from build123d import *

# Parameters (mm, degrees)
BOX017_W               = 5
BOX017_H               = 32.5
BOX017_DEPTH           = 5
BOX017_PITCH_ANGLE     = 45
BOX016_W               = 3
BOX016_H               = 32.5
BOX016_DEPTH           = 15
CYLINDER001_R          = 1.6
CYLINDER001_DEPTH      = 35
CYLINDER001_ROLL_ANGLE = 90
CYLINDER_R             = 1.6
CYLINDER_DEPTH         = 10
BOX006_W               = 10
BOX006_H               = 32.5
BOX006_DEPTH           = 10
BOX006_PITCH_ANGLE     = -10
BOX001_W               = 35
BOX001_H               = 32.5
BOX001_DEPTH           = 3
BOX002_W               = 35
BOX002_H               = 3
BOX002_DEPTH           = 3
BOX003_W               = 35
BOX003_H               = 3
BOX003_DEPTH           = 3
BOX004_W               = 35
BOX004_H               = 3
BOX004_DEPTH           = 3
BOX005_W               = 35
BOX005_H               = 3
BOX005_DEPTH           = 3
BOX007_W               = 9
BOX007_H               = 32.5
BOX007_DEPTH           = 13.5
BOX008_W               = 3
BOX008_H               = 3
BOX008_DEPTH           = 52
BOX009_W               = 3
BOX009_H               = 3
BOX009_DEPTH           = 52
BOX010_W               = 3
BOX010_H               = 3
BOX010_DEPTH           = 52
BOX011_W               = 3
BOX011_H               = 3
BOX011_DEPTH           = 52
BOX012_W               = 3
BOX012_H               = 32.5
BOX012_DEPTH           = 6.5
BOX013_W               = 30
BOX013_H               = 32.5
BOX013_DEPTH           = 3
BOX014_W               = 30
BOX014_H               = 3
BOX014_DEPTH           = 3
BOX015_W               = 30
BOX015_H               = 3
BOX015_DEPTH           = 3
BOX_W                  = 3
BOX_H                  = 32.5
BOX_DEPTH              = 42.5


with BuildPart() as cube017:
    # Box017 → Box017 (new body)
    with BuildSketch(Plane.XY):
        with Locations((2.5, 16.25)):
            Rectangle(BOX017_W, BOX017_H)
    extrude(amount=BOX017_DEPTH)


with BuildPart() as cube017_1:
    # Box017 pitch: moved
    add(cube017.part.rotate(Axis((0, 0, 0), (0, 1, 0)), BOX017_PITCH_ANGLE))


with BuildPart() as cube017_2:
    # Box017 placement: moved
    add(cube017_1.part.moved(Location((0, 0, 0.5))))


with BuildPart() as cube016:
    # Box016 → Box016 (new body)
    with BuildSketch(Plane.XY.offset(-14.5)):
        with Locations((1.5, 16.25)):
            Rectangle(BOX016_W, BOX016_H)
    extrude(amount=BOX016_DEPTH)


with BuildPart() as cylinder001:
    # Cylinder001 → Cylinder001 (new body)
    with BuildSketch(Plane.XY):
        Circle(CYLINDER001_R)
    extrude(amount=CYLINDER001_DEPTH)


with BuildPart() as cylinder001_1:
    # Cylinder001 roll: moved
    add(cylinder001.part.rotate(Axis((0, 0, 0), (1, 0, 0)), CYLINDER001_ROLL_ANGLE))


with BuildPart() as cylinder001_2:
    # Cylinder001 placement: moved
    add(cylinder001_1.part.moved(Location((-1.5, 33, 5))))


with BuildPart() as cylinder:
    # Cylinder → Cylinder (new body)
    with BuildSketch(Plane(origin=(-19, 16.25, -8), x_dir=(1, 0, 0), z_dir=(0, 0, 1))):
        Circle(CYLINDER_R)
    extrude(amount=CYLINDER_DEPTH)


with BuildPart() as cube006:
    # Box006 → Box006 (new body)
    with BuildSketch(Plane.XY):
        with Locations((5, 16.25)):
            Rectangle(BOX006_W, BOX006_H)
    extrude(amount=BOX006_DEPTH)


with BuildPart() as cube006_1:
    # Box006 pitch: moved
    add(cube006.part.rotate(Axis((0, 0, 0), (0, 1, 0)), BOX006_PITCH_ANGLE))


with BuildPart() as cube006_2:
    # Box006 placement: moved
    add(cube006_1.part.moved(Location((29, 0, 32))))


with BuildPart() as cube001:
    # Box001 → Box001 (new body)
    with BuildSketch(Plane.XY.offset(42.5)):
        with Locations((17.5, 16.25)):
            Rectangle(BOX001_W, BOX001_H)
    extrude(amount=BOX001_DEPTH)


with BuildPart() as cube002:
    # Box002 → Box002 (new body)
    with BuildSketch(Plane.XY.offset(45.5)):
        with Locations((17.5, 1.5)):
            Rectangle(BOX002_W, BOX002_H)
    extrude(amount=BOX002_DEPTH)


with BuildPart() as cube003:
    # Box003 → Box003 (new body)
    with BuildSketch(Plane(origin=(0, 29.5, 45.5), x_dir=(1, 0, 0), z_dir=(0, 0, 1))):
        with Locations((17.5, 1.5)):
            Rectangle(BOX003_W, BOX003_H)
    extrude(amount=BOX003_DEPTH)


with BuildPart() as cube004:
    # Box004 → Box004 (new body)
    with BuildSketch(Plane(origin=(0, 10, 45.5), x_dir=(1, 0, 0), z_dir=(0, 0, 1))):
        with Locations((17.5, 1.5)):
            Rectangle(BOX004_W, BOX004_H)
    extrude(amount=BOX004_DEPTH)


with BuildPart() as cube005:
    # Box005 → Box005 (new body)
    with BuildSketch(Plane(origin=(0, 19.5, 45.5), x_dir=(1, 0, 0), z_dir=(0, 0, 1))):
        with Locations((17.5, 1.5)):
            Rectangle(BOX005_W, BOX005_H)
    extrude(amount=BOX005_DEPTH)


with BuildPart() as cube007:
    # Box007 → Box007 (new body)
    with BuildSketch(Plane(origin=(-6, 0, -4), x_dir=(1, 0, 0), z_dir=(0, 0, 1))):
        with Locations((4.5, 16.25)):
            Rectangle(BOX007_W, BOX007_H)
    extrude(amount=BOX007_DEPTH)


with BuildPart() as cube008:
    # Box008 → Box008 (new body)
    with BuildSketch(Plane(origin=(-3, 0, -3.5), x_dir=(1, 0, 0), z_dir=(0, 0, 1))):
        with Locations((1.5, 1.5)):
            Rectangle(BOX008_W, BOX008_H)
    extrude(amount=BOX008_DEPTH)


with BuildPart() as cube009:
    # Box009 → Box009 (new body)
    with BuildSketch(Plane(origin=(-3, 29.5, -3.5), x_dir=(1, 0, 0), z_dir=(0, 0, 1))):
        with Locations((1.5, 1.5)):
            Rectangle(BOX009_W, BOX009_H)
    extrude(amount=BOX009_DEPTH)


with BuildPart() as cube010:
    # Box010 → Box010 (new body)
    with BuildSketch(Plane(origin=(-3, 19.5, -3.5), x_dir=(1, 0, 0), z_dir=(0, 0, 1))):
        with Locations((1.5, 1.5)):
            Rectangle(BOX010_W, BOX010_H)
    extrude(amount=BOX010_DEPTH)


with BuildPart() as cube011:
    # Box011 → Box011 (new body)
    with BuildSketch(Plane(origin=(-3, 10, -3.5), x_dir=(1, 0, 0), z_dir=(0, 0, 1))):
        with Locations((1.5, 1.5)):
            Rectangle(BOX011_W, BOX011_H)
    extrude(amount=BOX011_DEPTH)


with BuildPart() as cube012:
    # Box012 → Box012 (new body)
    with BuildSketch(Plane.XY.offset(-6.5)):
        with Locations((1.5, 16.25)):
            Rectangle(BOX012_W, BOX012_H)
    extrude(amount=BOX012_DEPTH)


with BuildPart() as cube013:
    # Box013 → Box013 (new body)
    with BuildSketch(Plane(origin=(-30, 0, -7), x_dir=(1, 0, 0), z_dir=(0, 0, 1))):
        with Locations((15, 16.25)):
            Rectangle(BOX013_W, BOX013_H)
    extrude(amount=BOX013_DEPTH)


with BuildPart() as cube014:
    # Box014 → Box014 (new body)
    with BuildSketch(Plane(origin=(-30, 0, -10), x_dir=(1, 0, 0), z_dir=(0, 0, 1))):
        with Locations((15, 1.5)):
            Rectangle(BOX014_W, BOX014_H)
    extrude(amount=BOX014_DEPTH)


with BuildPart() as cube015:
    # Box015 → Box015 (new body)
    with BuildSketch(Plane(origin=(-30, 29.5, -10), x_dir=(1, 0, 0), z_dir=(0, 0, 1))):
        with Locations((15, 1.5)):
            Rectangle(BOX015_W, BOX015_H)
    extrude(amount=BOX015_DEPTH)


with BuildPart() as cut004:
    # Box → Box (new body)
    with BuildSketch(Plane.XY):
        with Locations((1.5, 16.25)):
            Rectangle(BOX_W, BOX_H)
    extrude(amount=BOX_DEPTH)

    # Fusion: union Cube001, Cube002, Cube003, Cube004, Cube005, Cube007, Cube008, Cube009, Cube010, Cube011, Cube012, Cube013, Cube014, Cube015
    add(cube001.part)
    add(cube002.part)
    add(cube003.part)
    add(cube004.part)
    add(cube005.part)
    add(cube007.part)
    add(cube008.part)
    add(cube009.part)
    add(cube010.part)
    add(cube011.part)
    add(cube012.part)
    add(cube013.part)
    add(cube014.part)
    add(cube015.part)

    # Cut: cut Cube006
    add(cube006_2.part, mode=Mode.SUBTRACT)

    # Cut001: cut Cylinder
    add(cylinder.part, mode=Mode.SUBTRACT)

    # Cut002: cut Cylinder001
    add(cylinder001_2.part, mode=Mode.SUBTRACT)

    # Cut003: cut Cube016
    add(cube016.part, mode=Mode.SUBTRACT)

    # Cut004: cut Cube017
    add(cube017_2.part, mode=Mode.SUBTRACT)


solid = cut004.part
Could you check a few things on this model? Use its own coordinates, in mm. A direction names the side the tool comes from. Give positions to 0.01 mm unless a question says otherwise; leave off trailing zeros. Order: outer loops, then holes, each group sorted by start corner. A loop starts at its lowest first (then second) coordinate and runs counter-clockwise, first axis right, second up. Notation, with made-up numbers: (26.5, 66) -> (73.5, 66) arc R11 cw to (73.5, 81) -> close; hole circle Ø1 at (20, -39.75). An arc over 180 degrees is marked (long way). Answer in a Markdown table with one row per item. Add a question column.
Item 1: For faces 3 (the flat face through (-16, 16, -4)), 4 (the flat face through (0, 6, 27)), 5 (the flat face through (-15, 3, -9)), 6 (the flat face through (0, 16, -4)), which set-ups out of +Z, -Z, +X, -X, +Y, -Y let a thin tool reach every point of the face, with its end or its side?
Item 2: Imagine slicing it at B-B (y = 16.25). List the corners of the cut face in (x, z) for me.
Item 3: Please list where these lines run through material, in increasing order: probe 1 along Y at (x, z) = (-1.5, 31); probe 2 along Y at (x, z) = (-19, -5); probe 3 along X at (y, z) = (30.5, 5).
Item 4: We'd pull the mould along Y, two halves only. Please class faces 1 (the flat face through (1.5, 16, 2)), 2 (the flat face through (-1, 13, 38)): pulls with the +Y half, pulls with the -Y half, needs draft (parallel to the pull), parting line crosses it, or undercut.
Item 5: Imagine slicing it at A-A (x = -1.5). List the corners of the cut face in (y, z) for me, and give its area (3 significant figures).
Item 6: I'm going to push flat-ended pins straight in: P1, Ø4, axis at y = 23.5, z = 4, coming from the -X side; P2, Ø1.5, axis at y = 27, z = 13.5, coming from the -X side; P3, Ø1.9, axis at x = -19, y = 16.25, coming from the +Z side; P4, Ø8, axis at y = 14.5, z = 29, coming from the -X side. Where does each tip first touch, or does it pass through?
Item 7: Imagine slicing it at C-C (z = 5). List the corners of the cut face in (x, y) for me.
Item 8: Imagine slicing it at D-D (y = 25). List the corners of the cut face in (x, z) for me.
Result:
| question | item | result |
|---|---|---|
| 1 | face 3 | +Z, -X, +Y, -Y |
| 1 | face 4 | +Z, -X |
| 1 | face 5 | -Z, +X, -X |
| 1 | face 6 | -Z, +X, +Y, -Y |
| 2 | outline | (-30, -7) -> (-20.6, -7) -> (-20.6, -4) -> (-30, -4) -> close; (-17.4, -7) -> (0, -7) -> (0, 0.5) -> (3, 3.5) -> (3, 42.5) -> (30.96, 42.5) -> (35, 43.21) -> (35, 45.5) -> (0, 45.5) -> (0, 9.5) -> (-6, 9.5) -> (-6, -4) -> (-17.4, -4) -> close; hole circle Ø3.2 at (-1.5, 5) |
| 3 | probe 1 | 0 to 3, 10 to 13, 19.5 to 22.5, 29.5 to 32.5 |
| 3 | probe 2 | 0 to 14.65, 17.85 to 32.5 |
| 3 | probe 3 | -6 to -3.1, 0.1 to 3 |
| 4 | face 1 | needs draft |
| 4 | face 2 | undercut |
| 5 | outline | (0, -10) -> (3, -10) -> (3, -7) -> (29.5, -7) -> (29.5, -10) -> (32.5, -10) -> (32.5, 3.4) -> (0, 3.4) -> close; (0, 6.6) -> (32.5, 6.6) -> (32.5, 48.5) -> (29.5, 48.5) -> (29.5, 9.5) -> (22.5, 9.5) -> (22.5, 48.5) -> (19.5, 48.5) -> (19.5, 9.5) -> (13, 9.5) -> (13, 48.5) -> (10, 48.5) -> (10, 9.5) -> (3, 9.5) -> (3, 48.5) -> (0, 48.5) -> close |
| 5 | area | 918 mm2 |
| 6 | P1 | x = -6 |
| 6 | P2 | x = 0 |
| 6 | P3 | through |
| 6 | P4 | x = -3 |
| 7 | outline | (-6, 0) -> (-3.1, 0) -> (-3.1, 32.5) -> (-6, 32.5) -> close; (0.1, 0) -> (3, 0) -> (3, 32.5) -> (0.1, 32.5) -> close |
| 8 | outline | (-30, -7) -> (0, -7) -> (0, 0.5) -> (3, 3.5) -> (3, 42.5) -> (30.96, 42.5) -> (35, 43.21) -> (35, 45.5) -> (0, 45.5) -> (0, 9.5) -> (-6, 9.5) -> (-6, -4) -> (-30, -4) -> close; hole circle Ø3.2 at (-1.5, 5) |
